Input: part model. Units: mm. Frame: model coordinates. A direction names the side the tool comes from. Give positions to 0.01 mm unless a question says otherwise; leave off trailing zeros. Loops run counter-clockwise (first coordinate to the right, second up) from the corner with the lowest first, then second, coordinate; pieces in that order, holes last. Notation, with made-up numbers: M 89.25,-30 L 139.25,-30 A17 cw 139.25,-11 Z; hole C -10,56 d1. An arc over 180 degrees is marked long. Answer as a JSON object with one key per item and string values. Group by question number.
Autodesk Inventor part; units mm, degrees
ref_plane "YZ Plane" through (0, 0, 0) normal (1, 0, 0) x (0, 1, 0)
ref_plane "XZ Plane" through (0, 0, 0) normal (0, 1, 0) x (-1, 0, 0)
ref_plane "XY Plane" through (0, 0, 0) normal (0, 0, 1) x (1, 0, 0)
sketch "Sketch1" plane through (0, 0, 0) normal (0, 1, 0) x (-1, 0, 0)
  line L0 (12.25, 23.75) -> (-12.25, 23.75)
  line L1 (-12.25, 23.75) -> (-12.25, -23.75)
  line L2 (-12.25, -23.75) -> (12.25, -23.75)
  line L3 (12.25, -23.75) -> (12.25, 23.75)
  point P0 (0, 0)
  dimension "d0" = 12.25
  dimension "d1" = 12.25
  dimension "d2" = 23.75
  dimension "d3" = 23.75
extrude "Extrusion1" add sketch "Sketch1" along normal blind 5
sketch "Sketch2" plane through (0, 5, 0) normal (0, 1, 0) x (1, 0, 0)
  circle A0 centre (0, -22) radius 1.5
  circle A1 centre (0, 22) radius 1.5
  point P0 (0, 0)
  dimension "d6" = 3
  dimension "d7" = 3
  dimension "d8" = 22
  dimension "d9" = 22
  dimension "d10" = 0
  dimension "d11" = 0
extrude "Extrusion2" cut sketch "Sketch2" against normal up to surface (5 mm away)
sketch "Sketch4" plane through (0, 5, 0) normal (0, 1, 0) x (1, 0, 0)
  circle A0 centre (0, -22) radius 1.5
  circle A1 centre (0, 22) radius 1.5
  line L0 (-12.25, -23.75) -> (12.25, -23.75)
  line L1 (12.25, -23.75) -> (12.25, 23.75)
  line L2 (12.25, 23.75) -> (-12.25, 23.75)
  line L3 (-12.25, 23.75) -> (-12.25, -23.75)
  circle A2 centre (0, -22) radius 2
  circle A3 centre (0, 22) radius 2
  point P0 (0, 0)
  dimension "d14" = 4
  dimension "d15" = 4
extrude "Extrusion3" cut sketch "Sketch4" against normal blind 3 contours A2 L0 | L0 A2 | A3 L2 | L2 A3
sketch "Sketch5" plane through (0, 0, 0) normal (0, -1, 0) x (1, 0, 0)
  line L0 (-12.25, -23.75) -> (-12.25, 23.75)
  line L1 (-12.25, 23.75) -> (12.25, 23.75)
  line L2 (12.25, -23.75) -> (-12.25, -23.75)
  line L3 (10.15, 19.65) -> (-10.15, 19.65)
  line L4 (-10.15, 19.65) -> (-10.15, -19.65)
  line L5 (-10.15, -19.65) -> (10.15, -19.65)
  line L6 (10.15, -19.65) -> (10.15, 19.65)
  line L7 (12.25, 23.75) -> (12.25, -23.75)
  point P0 (0, 0)
  dimension "d20" = 4.1
  dimension "d21" = 4.1
  dimension "d22" = 2.1
  dimension "d23" = 2.1
extrude "Extrusion4" cut sketch "Sketch5" against normal blind 2 contours L6 L5 L4 L3
equation "\"d21\" = d20"
equation "\"d23\" = d22"
properties part number "Bottom"
1. Mould query, pull axis X, two halves, no side actions, for faces 4 (the cylindrical face through (-0.195, 1.014, -23.487)), 5 (the flat face through (-12.25, 2, 0)), 6 (the flat face through (12.25, 2, 0)), 7 (the flat face through (-10.15, 1, 0)). Classes: pulls with the +X half, pulls with the -X half, needs draft (parallel to the pull), parting line crosses it, or undercut.
2. Section D-D (x = -2.75). Output: boundary loops of the cut face in (y, z), then the cut area to 3 significant figures.
3. Section B-B (x = 0). Output: boundary loops of the cut face in (y, z).
4. First-contact query: P1, Ø3.5, axis at x = 0, z = -22, coming from the +Y side; P2, Ø1.9, axis at x = 1, z = 21.5, coming from the +Y side; P3, Ø1.8, axis at x = 0, z = 22, coming from the -Y side; P4, Ø6, axis at x = -0.5, z = -5.5, coming from the -Y side. Flat tips, straight axial feed; report the tip coordinate or a pass-through.
5. Material intervals for L1, parallel to Z at x = 0, y = 0.5; L2, parallel to X at y = 0.8, z = 1; L3, parallel to X at y = 1.3, z = -22, sorted ascending.
6. Section A-A (z = -22). Output: boundary loops of the cut face in (x, y).
7. Section C-C (y = 0.7). Output: boundary loops of the cut face in (x, z).
8. Reachability of faces 1 (the cylindrical face through (0, 4, 20)), 2 (the flat face through (-11, 0, 0)), 3 (the flat face through (10.15, 1, 0)) from +Z, -Z, +X, -X, +Y, -Y: full face, straight path, thin tool, end or side. Return the list, or none.
Geometry results:
{
 "1": {"face 4": "undercut", "face 5": "pulls with the -X half", "face 6": "pulls with the +X half", "face 7": "undercut"},
 "2": {"outline": "M 0,-23.75 L 5,-23.75 L 5,23.75 L 0,23.75 L 0,19.65 L 2,19.65 L 2,-19.65 L 0,-19.65 Z", "area": "159 mm2"},
 "3": {"outline": "M 0,-23.75 L 2,-23.75 L 2,-23.5 L 0,-23.5 Z; M 0,-20.5 L 2,-20.5 L 2,-20 L 5,-20 L 5,20 L 2,20 L 2,20.5 L 0,20.5 L 0,19.65 L 2,19.65 L 2,-19.65 L 0,-19.65 Z; M 0,23.5 L 2,23.5 L 2,23.75 L 0,23.75 Z"},
 "4": {"P1": "y = 2", "P2": "y = 5", "P3": "through", "P4": "y = 2"},
 "5": {"L1": "-23.75 to -23.5, -20.5 to -19.65, 19.65 to 20.5, 23.5 to 23.75", "L2": "-12.25 to -10.15, 10.15 to 12.25", "L3": "-12.25 to -1.5, 1.5 to 12.25"},
 "6": {"outline": "M -12.25,0 L -1.5,0 L -1.5,2 L -2,2 L -2,5 L -12.25,5 Z; M 1.5,0 L 12.25,0 L 12.25,5 L 2,5 L 2,2 L 1.5,2 Z"},
 "7": {"outline": "M -12.25,-23.75 L 12.25,-23.75 L 12.25,23.75 L -12.25,23.75 Z; hole M -10.15,-19.65 L 10.15,-19.65 L 10.15,19.65 L -10.15,19.65 Z; hole C 0,-22 d3; hole C 0,22 d3"},
 "8": {"face 1": "+Y", "face 2": "+Z, -Z, +X, -X, -Y", "face 3": "-Y"}
}
